```python
from build123d import *

# Parameters (mm, degrees)
BOSS_EXTRUDE1_DEPTH     = 2
BOSS_EXTRUDE1_2_DEPTH   = 2
BOSS_EXTRUDE1_3_DEPTH   = 2
BOSS_EXTRUDE1_4_DEPTH   = 2
SKETCH1_R               = 9.5
SKETCH1_R_2             = 7.5625
BOSS_EXTRUDE1_5_DEPTH   = 2
BOSS_EXTRUDE2_START     = -2
SKETCH2_R               = 15
BOSS_EXTRUDE2_DEPTH     = 2
FILLET1_R               = 0.1
FILLET2_R               = 0.1
SKETCH4_R               = 16
BOSS_EXTRUDE3_DEPTH     = 0.5
SKETCH5_R               = 17.5
BOSS_EXTRUDE4_DEPTH     = 4
CUT_EXTRUDE2_DEPTH      = 26.154522456
CUT_EXTRUDE2_DEPTH_BACK = 26.154522456
SKETCH3_R               = 1.6
SKETCH6_R               = 2.1
CUT_EXTRUDE3_DEPTH      = 4
SKETCH7_R               = 2.6
CUT_EXTRUDE4_DEPTH      = 4
SKETCH8_R               = 6.75
MIDDLE_CUTOUT_DEPTH     = 7
CHAMFER1_SIZE           = 0.1
CUT_EXTRUDE6_START      = -2
SKETCH9_R               = 7.5625
CUT_EXTRUDE6_DEPTH      = 2
CHAMFER2_SIZE           = 0.3
CHAMFER2_SIZE2          = 0.824243226


with BuildPart() as part:
    # Sketch1 → Boss-Extrude1 (new body)
    with BuildSketch(Plane.XY):
        with BuildLine():
            ThreePointArc((5.795745748, 11.075167323), (6.469207051, 12.179609111), (7.456549067, 13.01537076))
            ThreePointArc((7.456549067, 13.01537076), (0, 15), (-7.456549067, 13.01537076))
            ThreePointArc((-7.456549067, 13.01537076), (-6.469207051, 12.179609111), (-5.795745748, 11.075167323))
            ThreePointArc((-5.795745748, 11.075167323), (0, 12.5), (5.795745748, 11.075167323))
        make_face()
    extrude(amount=BOSS_EXTRUDE1_DEPTH)



with BuildPart() as body_2:
    # Sketch1 → Boss-Extrude1 2 (new body)
    with BuildSketch(Plane.XY):
        with BuildLine():
            ThreePointArc((13.01537076, -7.456549067), (14.495353762, -3.858071967), (15, 0))
            ThreePointArc((15, 0), (14.495353762, 3.858071967), (13.01537076, 7.456549067))
            ThreePointArc((13.01537076, 7.456549067), (12.179609111, 6.469207051), (11.075167323, 5.795745748))
            ThreePointArc((11.075167323, 5.795745748), (12.5, 0), (11.075167323, -5.795745748))
            ThreePointArc((11.075167323, -5.795745748), (12.179609111, -6.469207051), (13.01537076, -7.456549067))
        make_face()
    extrude(amount=BOSS_EXTRUDE1_2_DEPTH)


with BuildPart() as body_3:
    # Sketch1 → Boss-Extrude1 3 (new body)
    with BuildSketch(Plane.XY):
        with BuildLine():
            ThreePointArc((-7.456549067, -13.01537076), (0, -15), (7.456549067, -13.01537076))
            ThreePointArc((7.456549067, -13.01537076), (6.469207051, -12.179609111), (5.795745748, -11.075167323))
            ThreePointArc((5.795745748, -11.075167323), (0, -12.5), (-5.795745748, -11.075167323))
            ThreePointArc((-5.795745748, -11.075167323), (-6.469207051, -12.179609111), (-7.456549067, -13.01537076))
        make_face()
    extrude(amount=BOSS_EXTRUDE1_3_DEPTH)


with BuildPart() as body_4:
    # Sketch1 → Boss-Extrude1 4 (new body)
    with BuildSketch(Plane.XY):
        with BuildLine():
            ThreePointArc((-11.075167323, 5.795745748), (-12.179609111, 6.469207051), (-13.01537076, 7.456549067))
            ThreePointArc((-13.01537076, 7.456549067), (-15, 0), (-13.01537076, -7.456549067))
            ThreePointArc((-13.01537076, -7.456549067), (-12.179609111, -6.469207051), (-11.075167323, -5.795745748))
            ThreePointArc((-11.075167323, -5.795745748), (-12.5, 0), (-11.075167323, 5.795745748))
        make_face()
    extrude(amount=BOSS_EXTRUDE1_4_DEPTH)


with BuildPart() as body_5:
    # Sketch1 → Boss-Extrude1 5 (new body)
    with BuildSketch(Plane.XY):
        Circle(SKETCH1_R)
        Circle(SKETCH1_R_2, mode=Mode.SUBTRACT)
    extrude(amount=BOSS_EXTRUDE1_5_DEPTH)


with BuildPart() as part_1:
    add(part.part)

    add(body_2.part)  # Boss-Extrude2 merges body 2

    add(body_3.part)  # Boss-Extrude2 merges body 3

    add(body_4.part)  # Boss-Extrude2 merges body 4

    add(body_5.part)  # Boss-Extrude2 merges body 5
    # Sketch2 → Boss-Extrude2 (add)
    with BuildSketch(Plane.XY.offset(BOSS_EXTRUDE2_START)):
        with Locations(Location((0, 0, 0), (0, 0, 150.191461703))):
            Circle(SKETCH2_R)
    extrude(amount=BOSS_EXTRUDE2_DEPTH)

    # Fillet1
    fillet1_edges = [part_1.edges().sort_by_distance(p)[0] for p in [
        (11.075167323, 5.795745748, 1),
        (11.075167323, -5.795745748, 1),
        (5.795745748, -11.075167323, 1),
        (-5.795745748, -11.075167323, 1),
        (-11.075167323, -5.795745748, 1),
        (-11.075167323, 5.795745748, 1),
        (5.795745748, 11.075167323, 1),
        (-5.795745748, 11.075167323, 1),
    ]]
    fillet(fillet1_edges, radius=FILLET1_R)

    # Fillet2
    fillet2_edges = [part_1.edges().sort_by_distance(p)[0] for p in [
        (6.504180663, 12.219925602, 2),
        (12.219925602, -6.504180663, 2),
        (-6.504180663, -12.219925602, 2),
        (-12.219925602, 6.504180663, 2),
        (-9.5, 0, 2),
        (0, -12.5, 2),
        (6.504180663, -12.219925602, 2),
        (5.779303749, -11.119440592, 2),
        (-5.779303749, -11.119440592, 2),
        (12.5, 0, 2),
        (12.219925602, 6.504180663, 2),
        (11.119440592, 5.779303749, 2),
        (11.119440592, -5.779303749, 2),
        (0, 12.5, 2),
        (-6.504180663, 12.219925602, 2),
        (-5.779303749, 11.119440592, 2),
        (5.779303749, 11.119440592, 2),
        (-12.5, 0, 2),
        (-12.219925602, -6.504180663, 2),
        (-11.119440592, -5.779303749, 2),
        (-11.119440592, 5.779303749, 2),
    ]]
    fillet(fillet2_edges, radius=FILLET2_R - 0.0001)  # a hair under: the kernel refuses the full size

    # Sketch4 → Boss-Extrude3 (add)
    with BuildSketch(Plane(origin=(0, 0, -2), x_dir=(-1, 0, 0), z_dir=(0, 0, -1))):
        Circle(SKETCH4_R)
    extrude(amount=BOSS_EXTRUDE3_DEPTH)

    # Sketch5 → Boss-Extrude4 (add)
    with BuildSketch(Plane(origin=(0, 0, -2.5), x_dir=(-1, 0, 0), z_dir=(0, 0, -1))):
        Circle(SKETCH5_R)
    extrude(amount=BOSS_EXTRUDE4_DEPTH)

    # Sketch3 → Cut-Extrude2 (cut, two sides: drawn at the far end of the back side and taken through both)
    with BuildSketch(Plane(origin=(0, 0, -2), x_dir=(-1, 0, 0), z_dir=(0, 0, -1)).offset(-CUT_EXTRUDE2_DEPTH_BACK)):
        with Locations((-9.192388155, 9.192388155)):
            Circle(SKETCH3_R)
        with Locations((9.192388155, 9.192388155)):
            Circle(SKETCH3_R)
        with Locations((9.192388155, -9.192388155)):
            Circle(SKETCH3_R)
        with Locations((-9.192388155, -9.192388155)):
            Circle(SKETCH3_R)
    extrude(amount=CUT_EXTRUDE2_DEPTH + CUT_EXTRUDE2_DEPTH_BACK, mode=Mode.SUBTRACT)

    # Sketch6 → Cut-Extrude3 (cut)
    with BuildSketch(Plane(origin=(0, 0, -6.5), x_dir=(-1, 0, 0), z_dir=(0, 0, -1))):
        with Locations((-9.192388155, 9.192388155)):
            Circle(SKETCH6_R)
        with Locations((9.192388155, 9.192388155)):
            Circle(SKETCH6_R)
        with Locations((9.192388155, -9.192388155)):
            Circle(SKETCH6_R)
        with Locations((-9.192388155, -9.192388155)):
            Circle(SKETCH6_R)
    extrude(amount=-CUT_EXTRUDE3_DEPTH, mode=Mode.SUBTRACT)

    # Sketch7 → Cut-Extrude4 (cut)
    with BuildSketch(Plane(origin=(0, 0, -6.5), x_dir=(-1, 0, 0), z_dir=(0, 0, -1))):
        with Locations((0, 13)):
            Circle(SKETCH7_R)
        with Locations((13, 0)):
            Circle(SKETCH7_R)
        with Locations((0, -13)):
            Circle(SKETCH7_R)
        with Locations((-13, 0)):
            Circle(SKETCH7_R)
    extrude(amount=-CUT_EXTRUDE4_DEPTH, mode=Mode.SUBTRACT)

    # Sketch8 → Middle Cutout (cut)
    with BuildSketch(Plane.XY):
        Circle(SKETCH8_R)
    extrude(amount=-MIDDLE_CUTOUT_DEPTH, mode=Mode.SUBTRACT)

    # Chamfer1
    chamfer1_edges = [part_1.edges().sort_by_distance(p)[0] for p in [
        (17.5, 0, -6.5),
    ]]
    chamfer(chamfer1_edges, length=CHAMFER1_SIZE)

    # Sketch9 → Cut-Extrude6 (cut)
    with BuildSketch(Plane.XY.offset(CUT_EXTRUDE6_START)):
        Circle(SKETCH9_R)
    extrude(amount=CUT_EXTRUDE6_DEPTH, mode=Mode.SUBTRACT)

    # Chamfer2
    chamfer2_edges = [part_1.edges().sort_by_distance(p)[0] for p in [
        (17.5, 0, -2.5),
    ]]
    chamfer2_side = [part_1.faces().sort_by_distance(p)[0] for p in [
        (17.005025253, 0, -2.5),
    ]]
    chamfer(chamfer2_edges, length=CHAMFER2_SIZE, length2=CHAMFER2_SIZE2, reference=chamfer2_side[0])


solid = part_1.part
```
The model under review builds one solid part; all positions refer to its coordinate system, in mm. A direction names the side the tool comes from. Round coordinates to 2 decimals unless told otherwise and drop trailing zeros. Loops run counter-clockwise (first coordinate to the right, second up) from the corner with the lowest first, then second, coordinate; pieces in that order, holes last. Notation, with made-up numbers: (69, 83.5) -> (112, 83.5) arc R20 ccw to (112, 96.5) -> close; hole circle Ø9 at (26.25, -19.75). An arc over 180 degrees is marked (long way). Answer as a JSON object with one key per item and string values. Group by question number.
1) We need section A-A on z = -5.75. Give the number of separate pieces and of enclosed holes in the cut face, then the cut area to 3 significant figures.
2) Mouldability with a two-part tool opening along X and no side actions: class faces 1 (the face through (6.493, 12.207, 0.937)), 2 (the face through (13.887, -10.648, -4.841)), 3 (the face through (0, -13, -2.5)) as released by +X, released by -X, zero draft, split by the parting line, or undercut.
3) We need section B-B on z = -1.5. Write out the cut boundary in (x, y) (1 decimal).
4) For pin 1 Ø2 at (y, z) = (4, -2.5) entering from -X; pin 2 Ø5 at (y, z) = (12.5, -4) entering from -X; pin 3 Ø2 at (x, y) = (-10, -9) entering from -Z, all flat-tipped, find the tip position at first contact; note any pin that passes through.
5) For faces 4 (the face through (0.56, -15.54, -4.53)), 5 (the face through (-6.516, 12.233, 0.937)), 6 (the face through (-5, 5, -2)), 7 (the face through (12.207, -6.493, 0.937)), 8 (the face through (-12.207, 6.493, 0.937)), list the 3-axis set-ups (+Z, -Z, +X, -X, +Y, -Y) from which the entire face can be reached by the end or side of a thin tool; tool diameter is ignored.
6) For line 1 (Y direction, x = -1.5, z = -4.75); line 2 (Y direction, x = -3, z = 1); line 3 (X direction, y = -7, z = 1.5), list the stretches that pass through material, from the lowest coordinate up. Write a range as [from, to].
Result set:
{
 "1": {"separate pieces": "1", "enclosed holes": "9", "area": "679 mm²"},
 "2": {"face 1": "released by +X", "face 2": "split by the parting line", "face 3": "undercut"},
 "3": {"outline": "circle Ø30 at (0, 0); hole circle Ø3.2 at (-9.2, -9.2); hole circle Ø3.2 at (-9.2, 9.2); hole circle Ø15.1 at (0, 0); hole circle Ø3.2 at (9.2, -9.2); hole circle Ø3.2 at (9.2, 9.2)"},
 "4": {"pin 1": "x = -17.16", "pin 2": "x = -14.36", "pin 3": "z = -2.5"},
 "5": {"face 4": "-Z", "face 5": "+Z, -X", "face 6": "+Z", "face 7": "+Z, -Y", "face 8": "+Z, +Y"},
 "6": {"line 1": "[-17.44, -15.12], [-10.88, -6.58], [6.58, 10.88], [15.12, 17.44]", "line 2": "[-14.7, -12.13], [-9.01, -6.94], [6.94, 9.01], [12.13, 14.7]", "line 3": "[-13.27, -12.7], [-6.42, -2.86], [2.86, 6.42], [12.7, 13.27]"}
}
